Verification items for the finished model (mm, model axes). A direction names the side the tool comes from. Round coordinates to 2 decimals unless told otherwise and drop trailing zeros. Write each loop counter-clockwise with the first axis right and the second up, starting at its lowest first coordinate (ties: lowest second). Pieces come first, ordered by that corner, then holes. Notation, with made-up numbers: (54.5, 29.5) - (78.5, 29.5) arc R31 cw to (78.5, 67.5) - close; hole circle Ø8 at (27.25, -2). An arc over 180 degrees is marked (long way). Answer as a JSON object with one key per item and string values.
```python
from build123d import *

# Parameters (mm, degrees)
SKETCH2_R               = 3
SKETCH2_R_2             = 1.7
BOSS_EXTRUDE1_DEPTH     = 5
BOSS_EXTRUDE1_2_DEPTH   = 5
BOSS_EXTRUDE1_3_DEPTH   = 5
BOSS_EXTRUDE1_4_DEPTH   = 5
SKETCH3_W               = 56
SKETCH3_H               = 38.9
SKETCH3_R               = 1.7
BOSS_EXTRUDE2_DEPTH     = 4
FILLET1_R               = 5
CUT_EXTRUDE2_START      = 4
CUT_EXTRUDE2_DEPTH      = 2.5
CUT_EXTRUDE3_DEPTH      = 2.5
SKETCH5_R               = 3
SKETCH5_R_2             = 1.7
BOSS_EXTRUDE3_DEPTH     = 5
SKETCH5_2_R             = 1.7
CUT_EXTRUDE4_DEPTH      = 35.45725613
CUT_EXTRUDE5_DEPTH      = 2.5
CHAMFER1_SIZE           = 1
CHAMFER2_SIZE           = 1
CUT_EXTRUDE6_DEPTH      = 35.907771341
CUT_EXTRUDE6_DEPTH_BACK = 35.907771341
SKETCH7_W               = 7.5
SKETCH7_H               = 26
FILLET3_R               = 1


with BuildPart() as part:
    # Sketch2 → Boss-Extrude1 (new body)
    with BuildSketch(Plane(origin=(0, 0, 0), x_dir=(1, 0, 0), z_dir=(0, 1, 0))):
        with Locations(Location((-25, 7.5, 0), (0, 0, 270))):
            Circle(SKETCH2_R)
        with Locations(Location((-25, 7.5, 0), (0, 0, 270))):
            Circle(SKETCH2_R_2, mode=Mode.SUBTRACT)
    extrude(amount=BOSS_EXTRUDE1_DEPTH)



with BuildPart() as body_2:
    # Sketch2 → Boss-Extrude1 2 (new body)
    with BuildSketch(Plane(origin=(0, 0, 0), x_dir=(1, 0, 0), z_dir=(0, 1, 0))):
        with Locations(Location((-25, -7.5, 0), (0, 0, 270))):
            Circle(SKETCH2_R)
        with Locations(Location((-25, -7.5, 0), (0, 0, 270))):
            Circle(SKETCH2_R_2, mode=Mode.SUBTRACT)
    extrude(amount=BOSS_EXTRUDE1_2_DEPTH)


with BuildPart() as body_3:
    # Sketch2 → Boss-Extrude1 3 (new body)
    with BuildSketch(Plane(origin=(0, 0, 0), x_dir=(1, 0, 0), z_dir=(0, 1, 0))):
        with Locations(Location((25, -7.5, 0), (0, 0, 270))):
            Circle(SKETCH2_R)
        with Locations(Location((25, -7.5, 0), (0, 0, 270))):
            Circle(SKETCH2_R_2, mode=Mode.SUBTRACT)
    extrude(amount=BOSS_EXTRUDE1_3_DEPTH)


with BuildPart() as body_4:
    # Sketch2 → Boss-Extrude1 4 (new body)
    with BuildSketch(Plane(origin=(0, 0, 0), x_dir=(1, 0, 0), z_dir=(0, 1, 0))):
        with Locations(Location((25, 7.5, 0), (0, 0, 270))):
            Circle(SKETCH2_R)
        with Locations(Location((25, 7.5, 0), (0, 0, 270))):
            Circle(SKETCH2_R_2, mode=Mode.SUBTRACT)
    extrude(amount=BOSS_EXTRUDE1_4_DEPTH)


with BuildPart() as part_1:
    add(part.part)

    add(body_2.part)  # Boss-Extrude2 merges body 2

    add(body_3.part)  # Boss-Extrude2 merges body 3

    add(body_4.part)  # Boss-Extrude2 merges body 4
    # Sketch3 → Boss-Extrude2 (add)
    with BuildSketch(Plane(origin=(0, 0, 0), x_dir=(1, 0, 0), z_dir=(0, 1, 0))):
        Rectangle(SKETCH3_W, SKETCH3_H)
        with Locations(Location((-25, 7.5, 0), (0, 0, 270))):
            Circle(SKETCH3_R, mode=Mode.SUBTRACT)
        with Locations(Location((25, 7.5, 0), (0, 0, 270))):
            Circle(SKETCH3_R, mode=Mode.SUBTRACT)
        with Locations(Location((25, -7.5, 0), (0, 0, 270))):
            Circle(SKETCH3_R, mode=Mode.SUBTRACT)
        with Locations(Location((-25, -7.5, 0), (0, 0, 270))):
            Circle(SKETCH3_R, mode=Mode.SUBTRACT)
    extrude(amount=BOSS_EXTRUDE2_DEPTH)

    # Fillet1
    fillet1_edges = [part_1.edges().sort_by_distance(p)[0] for p in [
        (28, 2, 19.45),
        (28, 2, -19.45),
        (-28, 2, -19.45),
        (-28, 2, 19.45),
    ]]
    fillet(fillet1_edges, radius=FILLET1_R)

    # Sketch1 → Cut-Extrude2 (cut)
    with BuildSketch(Plane(origin=(0, 0, 0), x_dir=(1, 0, 0), z_dir=(0, 1, 0)).offset(CUT_EXTRUDE2_START)):
        Polygon((13.620101013, 19.45), (15.6, 17.470101013), (15.6, -19.45), (-15.6, -19.45), (-15.6, 17.470101013), (-13.620101013, 19.45), align=None)
    extrude(amount=-CUT_EXTRUDE2_DEPTH, mode=Mode.SUBTRACT)

    # Sketch4 → Cut-Extrude3 (cut)
    with BuildSketch(Plane(origin=(0, 4, 0), x_dir=(1, 0, 0), z_dir=(0, 1, 0))):
        Polygon((-16.1, -19.95), (16.1, -19.95), (16.1, 17.677207794), (13.827207794, 19.95), (-13.827207794, 19.95), (-16.1, 17.677207794), align=None)
    extrude(amount=-CUT_EXTRUDE3_DEPTH, mode=Mode.SUBTRACT)

    # Sketch5 → Boss-Extrude3 (add)
    # profile 1 of 4: a face of its own
    with BuildSketch(Plane(origin=(0, 4, 0), x_dir=(1, 0, 0), z_dir=(0, 1, 0))):
        with Locations(Location((-21.5, 15, 0), (0, 0, 90))):
            Circle(SKETCH5_R)
        with Locations(Location((-21.5, 15, 0), (0, 0, 270))):
            Circle(SKETCH5_R_2, mode=Mode.SUBTRACT)
    # profile 2 of 4: a face of its own
    with BuildSketch(Plane(origin=(0, 4, 0), x_dir=(1, 0, 0), z_dir=(0, 1, 0))):
        with Locations(Location((21.5, 15, 0), (0, 0, 90))):
            Circle(SKETCH5_R)
        with Locations(Location((21.5, 15, 0), (0, 0, 270))):
            Circle(SKETCH5_R_2, mode=Mode.SUBTRACT)
    # profile 3 of 4: a face of its own
    with BuildSketch(Plane(origin=(0, 4, 0), x_dir=(1, 0, 0), z_dir=(0, 1, 0))):
        with Locations(Location((21.5, -15, 0), (0, 0, 90))):
            Circle(SKETCH5_R)
        with Locations(Location((21.5, -15, 0), (0, 0, 270))):
            Circle(SKETCH5_R_2, mode=Mode.SUBTRACT)
    # profile 4 of 4: a face of its own
    with BuildSketch(Plane(origin=(0, 4, 0), x_dir=(1, 0, 0), z_dir=(0, 1, 0))):
        with Locations(Location((-21.5, -15, 0), (0, 0, 90))):
            Circle(SKETCH5_R)
        with Locations(Location((-21.5, -15, 0), (0, 0, 270))):
            Circle(SKETCH5_R_2, mode=Mode.SUBTRACT)
    extrude(amount=BOSS_EXTRUDE3_DEPTH)

    # Sketch5<2> → Cut-Extrude4 (cut, through all)
    with BuildSketch(Plane(origin=(0, 4, 0), x_dir=(1, 0, 0), z_dir=(0, 1, 0))):
        with Locations(Location((-21.5, 15, 0), (0, 0, 270))):
            Circle(SKETCH5_2_R)
        with Locations(Location((21.5, 15, 0), (0, 0, 270))):
            Circle(SKETCH5_2_R)
        with Locations(Location((21.5, -15, 0), (0, 0, 270))):
            Circle(SKETCH5_2_R)
        with Locations(Location((-21.5, -15, 0), (0, 0, 270))):
            Circle(SKETCH5_2_R)
    extrude(amount=-CUT_EXTRUDE4_DEPTH, mode=Mode.SUBTRACT)

    # Sketch6 → Cut-Extrude5 (cut)
    with BuildSketch(Plane.XZ):
        Polygon((-19.970021787, 12.35), (-18.440043573, 15), (-19.970021787, 17.65), (-23.029978213, 17.65), (-24.559956427, 15), (-23.029978213, 12.35), align=None)
        Polygon((23.029978213, 12.35), (24.559956427, 15), (23.029978213, 17.65), (19.970021787, 17.65), (18.440043573, 15), (19.970021787, 12.35), align=None)
        Polygon((24.559956427, -15), (23.029978213, -12.35), (19.970021787, -12.35), (18.440043573, -15), (19.970021787, -17.65), (23.029978213, -17.65), align=None)
        Polygon((-18.440043573, -15), (-19.970021787, -12.35), (-23.029978213, -12.35), (-24.559956427, -15), (-23.029978213, -17.65), (-19.970021787, -17.65), align=None)
    extrude(amount=-CUT_EXTRUDE5_DEPTH, mode=Mode.SUBTRACT)

    # Chamfer1
    chamfer1_edges = [part_1.edges().sort_by_distance(p)[0] for p in [
        (-21.5, 4, 18),
    ]]
    chamfer(chamfer1_edges, length=CHAMFER1_SIZE)

    # Chamfer2
    chamfer2_edges = [part_1.edges().sort_by_distance(p)[0] for p in [
        (-21.5, 4, -12),
        (21.5, 4, -12),
        (21.5, 4, 18),
    ]]
    chamfer(chamfer2_edges, length=CHAMFER2_SIZE)

    # Sketch7 → Cut-Extrude6 (cut, two sides: drawn at the far end of the back side and taken through both)
    with BuildSketch(Plane(origin=(0, 1.5, 0), x_dir=(1, 0, 0), z_dir=(0, 1, 0)).offset(-CUT_EXTRUDE6_DEPTH_BACK)):
        with Locations((-13.55, 0)):
            Rectangle(SKETCH7_W, SKETCH7_H)
        with Locations((13.55, 0)):
            Rectangle(SKETCH7_W, SKETCH7_H)
    extrude(amount=CUT_EXTRUDE6_DEPTH + CUT_EXTRUDE6_DEPTH_BACK, mode=Mode.SUBTRACT)

    # Fillet3
    fillet3_edges = [part_1.edges().sort_by_distance(p)[0] for p in [
        (-17.3, 2, 13),
        (-9.8, 0.75, -13),
        (-17.3, 2, -13),
        (-9.8, 0.75, 13),
        (17.3, 2, -13),
        (9.8, 0.75, 13),
        (17.3, 2, 13),
        (9.8, 0.75, -13),
    ]]
    fillet(fillet3_edges, radius=FILLET3_R)


solid = part_1.part
```
1. Cross-section at C-C (x = 5.5). Record the boundary of the cut face in (y, z).
Completed:
{"outline": "(0, -19.45) - (1.5, -19.45) - (1.5, 19.45) - (0, 19.45) - close"}
2. Access from +Z, -Z, +X, -X, +Y, -Y to the whole of each face (thin tool, end or side, straight path). Record for faces 1 (the face through (-25, 5, -5.5)), 2 (the face through (21, 2.5, -13)), 3 (the face through (-23, 4, 0)).
Completed:
{"face 1": "+X, -X, +Y", "face 2": "-Y", "face 3": "+Y"}
3. Cross-section at A-A (y = 7.75). Record the boundary of the cut face in (x, z), plus the area to 3 significant figures.
Completed:
{"outline": "circle Ø6 at (-21.5, -15); circle Ø6 at (-21.5, 15); circle Ø6 at (21.5, -15); circle Ø6 at (21.5, 15); hole circle Ø3.4 at (-21.5, -15); hole circle Ø3.4 at (-21.5, 15); hole circle Ø3.4 at (21.5, -15); hole circle Ø3.4 at (21.5, 15)", "area": "76.8 mm^2"}
4. Cross-section at B-B (z = -2). Record the boundary of the cut face in (x, y).
Completed:
{"outline": "(-28, 0) - (-17.3, 0) - (-17.3, 4) - (-28, 4) - close; (-9.8, 0) - (9.8, 0) - (9.8, 1.5) - (-9.8, 1.5) - close; (17.3, 0) - (28, 0) - (28, 4) - (17.3, 4) - close"}
5. Go/stop test with flat-tipped pins: pin 1 (3 mm diameter, centred on x = 15, y = 6, fed in from -Z); pin 2 (2 mm diameter, centred on y = 3, z = 16, fed in from +X); pin 3 (3 mm diameter, centred on x = -26.5, z = -8.5, fed in from +Y); pin 4 (4.5 mm diameter, centred on x = -21.5, z = -15, fed in from -Y). Record where each tip stops, or that it passes through.
Completed:
{"pin 1": "passes through", "pin 2": "stops at x = 27.97", "pin 3": "stops at y = 5", "pin 4": "stops at y = 2.5"}
6. Mould release check, pull along Z, two halves, no side actions. Record for faces 4 (the face through (0, 1, 19.45)), 5 (the face through (22, 1, 17.65)), 6 (the face through (0, 0, 0)): released by +Z, released by -Z, zero draft, split by the parting line, or undercut.
Completed:
{"face 4": "released by +Z", "face 5": "undercut", "face 6": "zero draft"}
7. Material ranges on probe 1 along Z at (x, y) = (22.5, 2); probe 2 along X at (y, z) = (5.85, -15); probe 3 along X at (y, z) = (2.5, -3.5), recorded low to high. Write a range as from..to.
Completed:
{"probe 1": "z = -19.45..-17.65, -12.35..12.35, 17.65..19.45", "probe 2": "x = -24.5..-23.2, -19.8..-18.5, 18.5..19.8, 23.2..24.5", "probe 3": "x = -28..-17.3, 17.3..28"}
